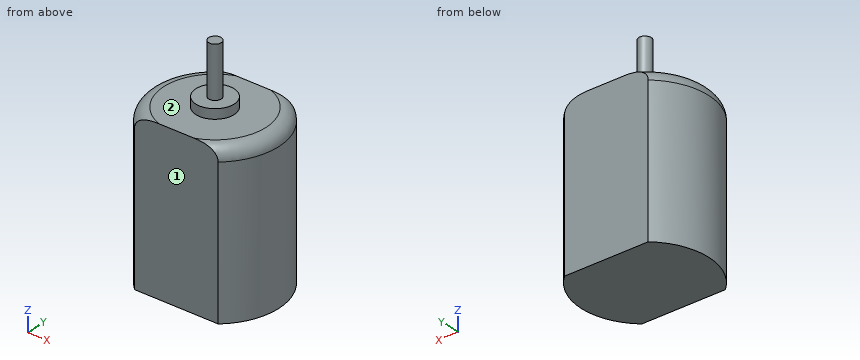
Autodesk Inventor part; units mm, degrees
ref_plane "YZ Plane" through (0, 0, 0) normal (1, 0, 0) x (0, 1, 0)
ref_plane "XZ Plane" through (0, 0, 0) normal (0, 1, 0) x (-1, 0, 0)
ref_plane "XY Plane" through (0, 0, 0) normal (0, 0, 1) x (1, 0, 0)
sketch "Sketch1" plane through (0, 0, 0) normal (0, 0, 1) x (1, 0, 0)
  circle A0 centre (0, 0) radius 10
  line L0 (-10, -7.5) -> (-10, 7.5)
  line L1 (-10, 7.5) -> (10, 7.5)
  line L2 (10, 7.5) -> (10, -7.5)
  line L3 (10, -7.5) -> (-10, -7.5)
  line L4 (-10, -7.5) -> (10, 7.5) construction
  line L5 (-10, 7.5) -> (10, -7.5) construction
  circle A1 centre (0, 0) radius 3
  circle A2 centre (0, 0) radius 1
  point P0 (-6.6144, -7.5)
  point P1 (6.6144, -7.5)
  point P2 (6.6144, 7.5)
  point P3 (-6.6144, 7.5)
  dimension "d0" = 20
  dimension "d1" = 15
  dimension "d2" = 6
  dimension "d3" = 2
extrude "Extrusion1" add sketch "Sketch1" along normal blind 1.5 contours A1
extrude "Extrusion2" add sketch "Sketch1" along normal blind 9.5 contours A2
extrude "Extrusion3" add sketch "Sketch1" against normal blind 25 contours A0 L3 L1 | A1 | A2
fillet "Fillet1" radius 2 2 edges at (-10, 0, 0) (10, 0, 0)
properties part number "Pumpe"
Geometry: final body of the model. Coordinates: model frame, mm. Face numbers are marked on the shaded views. A direction names the side the tool comes from. Coordinates: 2 decimals unless noted, no trailing zeros. Write each loop counter-clockwise with the first axis right and the second up, starting at its lowest first coordinate (ties: lowest second). Pieces come first, ordered by that corner, then holes. Notation, with made-up numbers: M 79,87.5 L 87,87.5 A9 ccw 87,96.5 Z; hole C 6.25,-35 d11. An arc over 180 degrees is marked long. Use CSV: the item, a comma, the result in double quotes. Start each with the question number.
1. Cut plane A-A on x = 0. Return the cut outline in (y, z).
2. First-contact query: P1, Ø1, axis at x = -2.5, z = 5.5, coming from the +Y side; P2, Ø6, axis at y = -4.5, z = -14, coming from the +X side; P3, Ø1.5, axis at y = 4, z = -10, coming from the -X side. Flat tips, straight axial feed; report the tip coordinate or a pass-through.
3. Ray query, probe 1 along Z at (x, y) = (-5.75, 2.75); probe 2 along Y at (x, z) = (-7.5, -9); probe 3 along Z at (x, y) = (0.75, 1.5). Return the intervals inside material, ascending.
4. Reachability of the marked faces 1 and 2 from +Z, -Z, +X, -X, +Y, -Y: full face, straight path, thin tool, end or side. Return the list, or none.
5. Cut plane C-C on z = -10. Return the cut outline in (x, y).
6. Cut plane B-B on y = 0. Return the cut outline in (x, z).
7. Cut plane D-D on z = -1. Return the cut outline in (x, y).
Entries:
1,outline,"M -7.5,-25 L 7.5,-25 L 7.5,0 L 3,0 L 3,1.5 L 1,1.5 L 1,9.5 L -1,9.5 L -1,1.5 L -3,1.5 L -3,0 L -7.5,0 Z"
2,P1,"through"
2,P2,"x = 9.89"
2,P3,"x = -9.46"
3,probe 1,"-25 to 0"
3,probe 2,"-6.61 to 6.61"
3,probe 3,"-25 to 1.5"
4,face 1,"+Z, -Z, +X, -X, -Y"
4,face 2,"+Z"
5,outline,"M -6.61,-7.5 L 6.61,-7.5 A10 ccw 6.61,7.5 L -6.61,7.5 A10 ccw Z"
6,outline,"M -10,-25 L 10,-25 L 10,-2 A2 ccw 8,0 L 3,0 L 3,1.5 L 1,1.5 L 1,9.5 L -1,9.5 L -1,1.5 L -3,1.5 L -3,0 L -8,0 A2 ccw -10,-2 Z"
7,outline,"M -6.2,-7.5 L 6.2,-7.5 A9.73 ccw 6.2,7.5 L -6.2,7.5 A9.73 ccw Z"
